Read the model definition and answer for the solid it produces. Units are mm, in the model's axes. A direction names the side the tool comes from. Coordinates: 2 decimals unless noted, no trailing zeros. Write each loop counter-clockwise with the first axis right and the second up, starting at its lowest first coordinate (ties: lowest second). Pieces come first, ordered by that corner, then holes. Notation, with made-up numbers: (20.5, -4.5) -> (66.5, -4.5) arc R24 ccw to (66.5, 19.5) -> close; hole circle Ø8 at (15, 85). An arc over 180 degrees is marked (long way). One line per item, written item: value. Start each with the question number.
1. Find section D-D, the plane z = -1.75. Write down the section's boundary in (x, y).
2. Find section B-B, the plane z = 5.65. Write down the section's boundary in (x, y), and give its area (3 significant figures).
3. For a pull along Z with two mould halves and no side action, classify faces 1 (the flat face through (0, 0, -10)), 2 (the flat face through (14, 17, 9.8)), 3 (the flat face through (-28, 9, -6.8)), 4 (the flat face through (-25, 8.15, 0)) as pulls with the +Z half, pulls with the -Z half, needs draft (parallel to the pull), parting line crosses it, or undercut.
4. Find section C-C, the plane y = 14. Write down the section's boundary in (x, z).
5. For faces 5 (the flat face through (28, 9, -6.8)), 6 (the flat face through (19.95, 12, 0)), 7 (the flat face through (-28, 9, -4.5)), 8 (the flat face through (-19.95, -5, 0)), determine the directions among +Z, -Z, +X, -X, +Y, -Y from which every point of the face is accessible in a straight line to the end or side of a thin tool.
6. Find section A-A, the plane x = 24.95. Write down the section's boundary in (y, z), and give its area (3 significant figures).
7. Given P1, Ø4, axis at x = 24.95, z = 5.65, coming from the +Y side; P2, Ø2, axis at y = 7, z = -0.5, coming from the -X side; P3, Ø0.6, axis at y = 12, z = 3.5, coming from the +X side; P4, Ø10.5, axis at x = -25.5, z = -5, coming from the +Y side, each flat-ended and moving along its own axis, determine where each tip first touches the part or whether it passes through.
8. Consider line 1 along Z through (x, y) = (-24.95, 9.6); line 2 along Z through (x, y) = (24, 10); line 3 along Y through (x, z) = (-23.5, 2). Determine where each line is inside the solid, lowest interval first.
```python
from build123d import *

# Parameters (mm, degrees)
SKETCH1_W           = 39.9
SKETCH1_H           = 20
BOSS_EXTRUDE1_DEPTH = 18.25
SKETCH2_W           = 20
SKETCH2_H           = 2.6
BOSS_EXTRUDE2_DEPTH = 9.7
CUT_EXTRUDE1_DEPTH  = 41.15202361
BOSS_EXTRUDE3_DEPTH = 19.8
CUT_EXTRUDE2_REACH  = 44.663
CUT_EXTRUDE4_DEPTH  = 0.2
CUT_EXTRUDE5_REACH  = 42.152


with BuildPart() as part:
    # Sketch1 → Boss-Extrude1 (new, symmetric)
    with BuildSketch(Plane(origin=(0, 0, 0), x_dir=(1, 0, 0), z_dir=(0, 1, 0))):
        Rectangle(SKETCH1_W, SKETCH1_H)
    extrude(amount=BOSS_EXTRUDE1_DEPTH, both=True)

    # Sketch2 → Boss-Extrude2 (add)
    with BuildSketch(Plane(origin=(19.95, 0, 0), x_dir=(0, 0, -1), z_dir=(1, 0, 0))):
        with Locations((0, 9.45)):
            Rectangle(SKETCH2_W, SKETCH2_H)
    boss_extrude2 = extrude(amount=BOSS_EXTRUDE2_DEPTH)

    # Sketch3 → Cut-Extrude1 (cut, through all)
    with BuildSketch(Plane.XY.offset(10)):
        Polygon((19.95, 12.75), (3.864292058, 18.25), (19.95, 18.25), align=None)
    extrude(amount=-CUT_EXTRUDE1_DEPTH, mode=Mode.SUBTRACT)

    # Sketch5 → Boss-Extrude3 (add)
    with BuildSketch(Plane.XY.offset(10)):
        Polygon((3.864292058, 18.25), (16.853835423, 18.25), (18.057563772, 13.397058824), align=None)
    extrude(amount=-BOSS_EXTRUDE3_DEPTH)

    # Sketch7 → Cut-Extrude2 (cut, up to next)
    with BuildSketch(Plane(origin=(0, 10.75, 0), x_dir=(1, 0, 0), z_dir=(0, 1, 0)), mode=Mode.PRIVATE) as cut_extrude2_sk1:
        with BuildLine():
            Line((29.65, 6.8), (27.281844763, 6.8))
            ThreePointArc((27.281844763, 6.8), (22.35, 5.65), (27.281844763, 4.5))
            Line((27.281844763, 4.5), (29.65, 4.5))
            Line((29.65, 4.5), (29.65, 6.8))
        make_face()
    cut_extrude2_tool1 = extrude(cut_extrude2_sk1.sketch, amount=-CUT_EXTRUDE2_REACH, mode=Mode.PRIVATE) & part.part
    # Sketch7 → Cut-Extrude2 (cut, up to next)
    with BuildSketch(Plane(origin=(0, 10.75, 0), x_dir=(1, 0, 0), z_dir=(0, 1, 0)), mode=Mode.PRIVATE) as cut_extrude2_sk2:
        with BuildLine():
            Line((29.65, -6.8), (27.281844763, -6.8))
            ThreePointArc((27.281844763, -6.8), (22.35, -5.65), (27.281844763, -4.5))
            Line((27.281844763, -4.5), (29.65, -4.5))
            Line((29.65, -4.5), (29.65, -6.8))
        make_face()
    cut_extrude2_tool2 = extrude(cut_extrude2_sk2.sketch, amount=-CUT_EXTRUDE2_REACH, mode=Mode.PRIVATE) & part.part
    cut_extrude2_1 = cut_extrude2_tool1.solids().sort_by_distance((25.640431, 10.75, -5.65))[0]
    add(cut_extrude2_1, mode=Mode.SUBTRACT)
    cut_extrude2_2 = cut_extrude2_tool2.solids().sort_by_distance((25.640431, 10.75, 5.65))[0]
    add(cut_extrude2_2, mode=Mode.SUBTRACT)
    cut_extrude2 = cut_extrude2_1 + cut_extrude2_2  # Cut-Extrude2 as one shape, for the pattern or mirror that repeats it

    # Sketch9 → Cut-Extrude4 (cut)
    with BuildSketch(Plane.XY.offset(10)):
        Polygon((16.853835423, 18.25), (3.864292058, 18.25), (18.057563772, 13.397058824), align=None)
    extrude(amount=-CUT_EXTRUDE4_DEPTH, mode=Mode.SUBTRACT)

    # Sketch10 → Cut-Extrude5 (cut, up to next)
    with BuildSketch(Plane(origin=(0, 0, -10), x_dir=(-1, 0, 0), z_dir=(0, 0, -1)), mode=Mode.PRIVATE) as cut_extrude5_sk1:
        Polygon((16.837123517, 18.25), (19.95, 16.25), (19.95, 18.25), align=None)
    cut_extrude5_tool1 = extrude(cut_extrude5_sk1.sketch, amount=-CUT_EXTRUDE5_REACH, mode=Mode.PRIVATE) & part.part
    add(cut_extrude5_tool1.solids().sort_by_distance((-18.912375, 17.583333, -10))[0], mode=Mode.SUBTRACT)

    # Mirror1: Boss-Extrude2, Cut-Extrude2 across plane
    add(boss_extrude2.mirror(Plane(origin=(0, 0, 0), x_dir=(0, 0, 1), z_dir=(1, 0, 0))))
    add(cut_extrude2.mirror(Plane(origin=(0, 0, 0), x_dir=(0, 0, 1), z_dir=(1, 0, 0))), mode=Mode.SUBTRACT)


solid = part.part
```
Answer block:
1. outline: (-29.65, 8.15) -> (-19.95, 8.15) -> (-19.95, -18.25) -> (19.95, -18.25) -> (19.95, 8.15) -> (29.65, 8.15) -> (29.65, 10.75) -> (19.95, 10.75) -> (19.95, 12.75) -> (18.06, 13.4) -> (16.85, 18.25) -> (-16.84, 18.25) -> (-19.95, 16.25) -> (-19.95, 10.75) -> (-29.65, 10.75) -> close
2. outline: (-22.35, 8.15) -> (-19.95, 8.15) -> (-19.95, -18.25) -> (19.95, -18.25) -> (19.95, 8.15) -> (22.35, 8.15) -> (22.35, 10.75) -> (19.95, 10.75) -> (19.95, 12.75) -> (18.06, 13.4) -> (16.85, 18.25) -> (-16.84, 18.25) -> (-19.95, 16.25) -> (-19.95, 10.75) -> (-22.35, 10.75) -> close
2. area: 1,450 mm2
3. face 1: pulls with the -Z half
3. face 2: pulls with the +Z half
3. face 3: undercut
3. face 4: needs draft
4. outline: (-19.95, -10) -> (16.29, -10) -> (16.29, -9.8) -> (17.91, -9.8) -> (17.91, 9.8) -> (16.29, 9.8) -> (16.29, 10) -> (-19.95, 10) -> close
5. face 5: +X, +Y, -Y
5. face 6: +Z, -Z, +X, +Y
5. face 7: -X, +Y, -Y
5. face 8: +Z, -Z, -X, -Y
6. outline: (8.15, -10) -> (10.75, -10) -> (10.75, -8.25) -> (8.15, -8.25) -> close; (8.15, -3.05) -> (10.75, -3.05) -> (10.75, 3.05) -> (8.15, 3.05) -> close; (8.15, 8.25) -> (10.75, 8.25) -> (10.75, 10) -> (8.15, 10) -> close
6. area: 25.0 mm2
7. P1: passes through
7. P2: stops at x = -19.95
7. P3: stops at x = 19.95
7. P4: stops at y = 10.75
8. line 1: z = -10 to -8.25, -3.05 to 3.05, 8.25 to 10
8. line 2: z = -10 to -8.07, -3.23 to 3.23, 8.07 to 10
8. line 3: y = 8.15 to 10.75
